```python
from build123d import *

# Parameters (mm, degrees)
F0_W     = 101.6
F0_H     = 2095.5
F1_DEPTH = 6.35
F2_W     = 6.35
F2_H     = 2095.5
F3_DEPTH = 101.6


with BuildPart() as f1:
    # F0 (on Front) → F1 (new body)
    with BuildSketch(Plane.XZ):
        Polygon((0, 2197.1), (0, 2095.5), (101.6, 2095.5), (984.25, 2095.5), (1085.85, 2095.5), (1085.85, 2197.1), align=None)
        with Locations((50.8, 1047.75)):
            Rectangle(F0_W, F0_H)
        with Locations((1035.05, 1047.75)):
            Rectangle(F0_W, F0_H)
    extrude(amount=F1_DEPTH)

    # F2 (on face) → F3 (join)
    with BuildSketch(Plane.XZ.offset(6.35)):
        Polygon((0, 2101.85), (0, 2095.5), (95.25, 2095.5), (101.6, 2095.5), (984.25, 2095.5), (990.6, 2095.5), (1085.85, 2095.5), (1085.85, 2101.85), align=None)
        with Locations((98.425, 1047.75)):
            Rectangle(F2_W, F2_H)
        with Locations((987.425, 1047.75)):
            Rectangle(F2_W, F2_H)
    extrude(amount=F3_DEPTH)


solid = f1.part
```
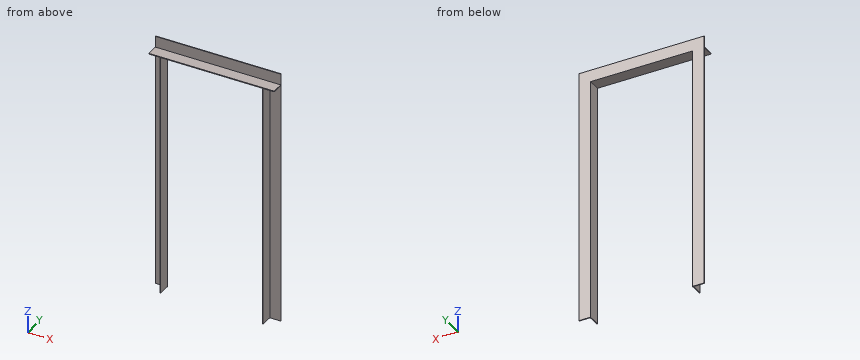
Work out the finished part from the listing and answer in its coordinate system (mm). Give positions to 0.01 mm unless a question says otherwise; leave off trailing zeros. Loops run counter-clockwise (first coordinate to the right, second up) from the corner with the lowest first, then second, coordinate; pieces in that order, holes last. Notation, with made-up numbers: M 78.25,78.25 L 121.25,78.25 A15 cw 121.25,96.25 Z; hole C 16,-16 d11. An arc over 180 degrees is marked long. One line per item, written item: value. Start each with the question number.
1. Find the intervals of material crossed by probe 1 along X at (y, z) = (-68.5, 378); probe 2 along Y at (x, z) = (1018, 1061); probe 3 along Z at (x, y) = (75.5, -29.5), in increasing order.
2. Find section B-B (y = -87). Give the vertices of the cut face in (x, z).
3. Find section D-D (x = 328). Give the vertices of the cut face in (y, z), and give its area (3 significant figures).
4. Each of these flat-tipped pins is pushed along its axis until it touches: P1, Ø4, axis at x = 889, y = -49, coming from the +Z side; P2, Ø4, axis at x = 836.5, y = -64, coming from the -Z side. Where does it stop, or does it pass through?
5. Find section C-C (x = 1018.5). Give the vertices of the cut face in (y, z).
6. Find section A-A (z = 1711). Give the vertices of the cut face in (x, y), and give its area (3 significant figures).
Reported:
1. probe 1: x = 95.25 to 101.6, 984.25 to 990.6
1. probe 2: y = -6.35 to 0
1. probe 3: z = 2095.5 to 2101.85
2. outline: M 0,2095.5 L 95.25,2095.5 L 95.25,0 L 101.6,0 L 101.6,2095.5 L 984.25,2095.5 L 984.25,0 L 990.6,0 L 990.6,2095.5 L 1085.85,2095.5 L 1085.85,2101.85 L 0,2101.85 Z
3. outline: M -107.95,2095.5 L 0,2095.5 L 0,2197.1 L -6.35,2197.1 L -6.35,2101.85 L -107.95,2101.85 Z
3. area: 1,290 mm²
4. P1: stops at z = 2101.85
4. P2: stops at z = 2095.5
5. outline: M -107.95,2095.5 L -6.35,2095.5 L -6.35,0 L 0,0 L 0,2197.1 L -6.35,2197.1 L -6.35,2101.85 L -107.95,2101.85 Z
6. outline: M 0,-6.35 L 95.25,-6.35 L 95.25,-107.95 L 101.6,-107.95 L 101.6,0 L 0,0 Z; M 984.25,-107.95 L 990.6,-107.95 L 990.6,-6.35 L 1085.85,-6.35 L 1085.85,0 L 984.25,0 Z
6. area: 2,580 mm²
